Geometry check sheet. Reference: the model listing, model coordinates, mm. A direction names the side the tool comes from. Give positions to 0.01 mm unless a question says otherwise; leave off trailing zeros. Order: outer loops, then holes, each group sorted by start corner. A loop starts at its lowest first (then second) coordinate and runs counter-clockwise, first axis right, second up. Notation, with made-up numbers: M -23,-33.5 L -8,-33.5 A27 ccw -8,-1.5 Z; hole C 88.5,71 d7. An arc over 180 degrees is marked long. Put each result on its own line as item: value. Start each with the question number.
Q1. Section check D-D on z = 14.5. Record the cut outline in (x, y).
Q2. Section check A-A on y = 30. Record the cut outline in (x, z).
Q3. Material ranges on L1, parallel to Z at x = 14, y = 2.25; L2, parallel to Y at x = 1.1, z = 36; L3, parallel to Y at x = 16.25, z = 31.5, recorded low to high.
Q4. Section check C-C on x = 18. Record the cut outline in (y, z).
Q5. Access from +Z, -Z, +X, -X, +Y, -Y to the whole of each face (thin tool, end or side, straight path). Record for faces 5 (the flat face through (3, 20, 21)), 6 (the flat face through (25, 2, 21)).
Q6. Mould release check, pull along Y, two halves, no side actions. Record for faces 1 (the cylindrical face through (1.479, 31.586, 5.792)), 2 (the cylindrical face through (1.48, 31.08, 34.82)), 3 (the flat face through (19, 3, 16)), 4 (the flat face through (10, 0, 16)): +Y half, -Y half, draft (parallel to the pull), parting line (faces both ways), or undercut.
Q7. Go/stop test with flat-tipped pins: pin 1 (6 mm diameter, centred on y = 20.5, z = 33.5, fed in from +X); pin 2 (1.5 mm diameter, centred on x = 4, y = 29.5, fed in from +Z); pin 3 (6.5 mm diameter, centred on x = 15, z = 28.5, fed in from +Y). Record where each tip stops, or that it passes through.
Q8. Section check B-B on z = 21. Record the cut outline in (x, y).
```python
from build123d import *

# Parameters (mm, degrees)
EXTRUDE_1_DEPTH     = 42
SKETCH_2_R          = 1.6
CUT_EXTRUDE_1_DEPTH = 26
SKETCH_3_R          = 6
CUT_EXTRUDE_2_DEPTH = 4


with BuildPart() as part:
    # ｽｹｯﾁ1 → ﾎﾞｽ - 押し出し1 (new body)
    with BuildSketch(Plane.XY):
        Polygon((0, 0), (0, 36), (3, 36), (3, 3), (25, 3), (25, 0), align=None)
    extrude(amount=EXTRUDE_1_DEPTH)

    # ｽｹｯﾁ2 → ｶｯﾄ - 押し出し1 (cut, through all)
    with BuildSketch(Plane.ZY):
        with Locations((36, 30)):
            Circle(SKETCH_2_R)
        with Locations((6, 30)):
            Circle(SKETCH_2_R)
    extrude(amount=-CUT_EXTRUDE_1_DEPTH, mode=Mode.SUBTRACT)

    # ｽｹｯﾁ3 → ｶｯﾄ - 押し出し2 (cut, through all)
    with BuildSketch(Plane(origin=(0, 3, 0), x_dir=(1, 0, 0), z_dir=(0, 1, 0))):
        with Locations((14, -21)):
            Circle(SKETCH_3_R)
    extrude(amount=-CUT_EXTRUDE_2_DEPTH, mode=Mode.SUBTRACT)


solid = part.part
```
Results found:
1. outline: M 0,0 L 25,0 L 25,3 L 3,3 L 3,36 L 0,36 Z
2. outline: M 0,0 L 3,0 L 3,4.4 L 0,4.4 Z; M 0,7.6 L 3,7.6 L 3,34.4 L 0,34.4 Z; M 0,37.6 L 3,37.6 L 3,42 L 0,42 Z
3. L1: z = 0 to 15, 27 to 42
3. L2: y = 0 to 28.4, 31.6 to 36
3. L3: y = 0 to 3
4. outline: M 0,0 L 3,0 L 3,16.53 L 0,16.53 Z; M 0,25.47 L 3,25.47 L 3,42 L 0,42 Z
5. face 5: +Z, -Z, +X, +Y
5. face 6: +Z, -Z, +X, +Y, -Y
6. face 1: undercut
6. face 2: undercut
6. face 3: +Y half
6. face 4: -Y half
7. pin 1: stops at x = 3
7. pin 2: passes through
7. pin 3: stops at y = 3
8. outline: M 0,0 L 8,0 L 8,3 L 3,3 L 3,36 L 0,36 Z; M 20,0 L 25,0 L 25,3 L 20,3 Z
